Autodesk Inventor part; units mm, degrees
ref_plane "YZ Plane" through (0, 0, 0) normal (1, 0, 0) x (0, 1, 0)
ref_plane "XZ Plane" through (0, 0, 0) normal (0, 1, 0) x (-1, 0, 0)
ref_plane "XY Plane" through (0, 0, 0) normal (0, 0, 1) x (1, 0, 0)
sketch "Sketch1" plane through (0, 0, 0) normal (0, 1, 0) x (-1, 0, 0)
  line L0 (0, 0) -> (105, 0)
  line L1 (105, 0) -> (105, -80)
  line L2 (105, -80) -> (0, -80)
  line L3 (0, -80) -> (0, 0)
  dimension "d0" = 105
  dimension "d1" = 80
extrude "Extrusion1" add sketch "Sketch1" along normal blind 5
sketch "Sketch2" plane through (0, 5, 0) normal (0, 1, 0) x (1, 0, 0)
  line L0 (0, 0) -> (0, 80)
  line L1 (-105, 80) -> (-105, 0)
  line L2 (0, 74) -> (-105, 74)
  line L3 (-105, 74) -> (-105, 7)
  line L4 (-105, 7) -> (0, 7)
  line L5 (0, 7) -> (0, 74)
  line L6 (-105, 0) -> (0, 0)
  line L7 (0, 80) -> (-105, 80)
  line L8 (-60, 7) -> (-60, 0)
  line L9 (-60, 7) -> (-65, 7)
  line L10 (-65, 7) -> (-65, 74)
  line L11 (-65, 74) -> (-60, 74)
  line L12 (-60, 74) -> (-60, 7)
  line L13 (-60, 64) -> (-65, 64)
  line L14 (-65, 64) -> (-65, 17)
  line L15 (-65, 17) -> (-60, 17)
  line L16 (-60, 17) -> (-60, 64)
  line L17 (0, 80) -> (-105, 80)
  line L18 (-105, 80) -> (-105, 0)
  line L19 (-105, 0) -> (0, 0)
  line L20 (0, 0) -> (0, 80)
  point P0 (-62.5, 74)
  point P1 (-62.5, 64)
  point P2 (-62.5, 7)
  point P3 (-62.5, 17)
  dimension "d4" = 7
  dimension "d5" = 6
  dimension "d7" = 45
  dimension "d8" = 5
  dimension "d9" = 10
  dimension "d10" = 10
extrude "Extrusion2" add sketch "Sketch2" along normal blind 25 contours L6 L1 L4 L8 | L2 L1 L7 L0 | L4 L10 L15 L12 | L12 L13 L10 L2
sketch "Sketch3" plane through (0, 30, 0) normal (0, 1, 0) x (1, 0, 0)
  line L0 (-100, 3.5) -> (-5, 3.5)
  line L1 (-5, 3.5) -> (-5, 77)
  line L2 (-5, 77) -> (-100, 77)
  line L3 (-100, 77) -> (-100, 3.5)
  line L4 (0, 80) -> (-105, 80)
  line L5 (-105, 0) -> (-60, 0)
  line L6 (-105, 74) -> (-105, 7)
  line L7 (0, 0) -> (0, 74)
  circle A0 centre (-100, 3.5) radius 1.5
  circle A1 centre (-100, 77) radius 1.5
  dimension "d13" = 3
  dimension "d14" = 3.5
  dimension "d15" = 5
  dimension "d16" = 5
  dimension "d17" = 3
  dimension "d20" = 3
extrude "Extrusion3" cut sketch "Sketch3" against normal blind 10 contours L3 A0 L0 | L0 A0 L3
extrude "Extrusion4" cut sketch "Sketch3" against normal blind 10 contours A1 L2 L3 | L3 L2 A1
pattern_linear "Rectangular Pattern2" count 4 spacing 12 along (1, 0, 0) of "Extrusion3"
pattern_linear "Rectangular Pattern3" count 9 spacing 12 along (1, 0, 0) of "Extrusion4"
sketch "Sketch4" plane through (0, 0, 0) normal (0, -1, 0) x (1, 0, 0)
  line L0 (-10, -12) -> (-80, -12)
  line L1 (-80, -12) -> (-80, -68)
  line L2 (-80, -68) -> (-10, -68)
  line L3 (-10, -68) -> (-10, -12)
  line L4 (0, -80) -> (-105, -80)
  line L5 (0, 0) -> (0, -80)
  line L6 (-80, -60) -> (-10, -68)
  line L7 (-10, -12) -> (-80, -20)
  circle A0 centre (-10, -12) radius 1.5
  circle A1 centre (-10, -68) radius 1.5
  circle A2 centre (-80, -20) radius 1.5
  circle A3 centre (-80, -60) radius 1.5
  point P0 (-80, -40)
  point P1 (-45, -68)
  point P2 (-11.5, -12)
  point P3 (-11.4903, -12.1703)
  dimension "d32" = 70
  dimension "d33" = 40
  dimension "d34" = 45
  dimension "d35" = 56
  dimension "d36" = 40
  dimension "d37" = 20
  dimension "d38" = 3
  dimension "d39" = 3
  dimension "d40" = 3
  dimension "d41" = 3
extrude "Extrusion5" cut sketch "Sketch4" against normal up to next contours L7 A0 L0 | L0 A0 L3 | L3 A0 L7 | A1 L2 L3 | L3 L6 A1 | A2 L1 L7 | L7 L1 A2 | L1 A2 | L2 A1 L6 | A3 L1 L6 | L6 L1 A3 | L1 A3
sketch "Sketch5" plane through (0, 5, 0) normal (0, 1, 0) x (1, 0, 0)
  line L0 (-105, 0) -> (0, 0)
  line L1 (0, 0) -> (-61.099, 0)
  line L2 (-61.099, 0) -> (-61.099, 7)
  line L3 (-61.099, 7) -> (0, 7)
  line L4 (0, 7) -> (0, 0)
  point P0 (-105, 7)
extrude "Extrusion6" add sketch "Sketch5" along normal blind 7.9
sketch "Sketch6" plane through (0, 0, -80) normal (0, 0, -1) x (-1, 0, 0)
  line L0 (97, 22) -> (79, 22)
  line L1 (79, 22) -> (79, 8)
  line L2 (79, 8) -> (97, 8)
  line L3 (97, 8) -> (97, 22)
  line L4 (0, 0) -> (105, 0)
  line L5 (0, 0) -> (0, 30)
  circle A0 centre (97, 8) radius 1.5
  circle A1 centre (97, 22) radius 1.5
  circle A2 centre (79, 22) radius 1.5
  circle A3 centre (79, 8) radius 1.5
  line L6 (105, 0) -> (105, 30)
  point P0 (79, 15)
  point P1 (105, 15)
  dimension "d46" = 15
  dimension "d47" = 14
  dimension "d48" = 18
  dimension "d50" = 3
  dimension "d51" = 3
  dimension "d52" = 3
  dimension "d53" = 3
  dimension "d56" = 8
extrude "Extrusion7" cut sketch "Sketch6" against normal up to surface (6 mm away) contours A2 L1 L0 | L0 L1 A2 | A1 L3 L0 | L0 L3 A1 | A3 L2 L1 | L1 L2 A3 | A0 L2 L3 | L3 L2 A0
sketch "Sketch7" plane through (0, 0, 0) normal (0, -1, 0) x (1, 0, 0)
  line L0 (-32, -27.5) -> (-48, -27.5)
  line L1 (-48, -27.5) -> (-48, -52.5)
  line L2 (-48, -52.5) -> (-32, -52.5)
  line L3 (-32, -52.5) -> (-32, -27.5)
  line L4 (0, 0) -> (0, -80)
  line L5 (-105, 0) -> (0, 0)
  line L6 (-46, -27.5) -> (-46, -52.5)
  line L7 (-44, -27.5) -> (-44, -52.5)
  circle A0 centre (-46, -29.75) radius 1.5
  circle A1 centre (-46, -50.25) radius 1.5
  circle A2 centre (-46, -50.25) radius 3.0104
  circle A3 centre (-46, -29.75) radius 3.0104
  line L8 (-42.9896, -50.25) -> (-42.9896, -52.5)
  line L9 (-42.9896, -29.75) -> (-42.9896, -27.5)
  point P0 (-40, -52.5)
  point P1 (-32, -40)
  point P2 (-46, -40)
  point P3 (-48, -40)
  point P4 (-46, -32.7604)
  point P5 (-46, -47.2396)
  dimension "d57" = 40
  dimension "d58" = 40
  dimension "d59" = 25
  dimension "d60" = 16
  dimension "d62" = 2
  dimension "d63" = 4
  dimension "d64" = 3
  dimension "d65" = 2.25
  dimension "d66" = 2.25
  dimension "d67" = 3
extrude "Extrusion8" cut sketch "Sketch7" against normal up to surface (5 mm away) contours L3 L2 L8 A2 L7 A3 L9 L0 | L7 A2 L6 A3 | A0 L6 | L6 A0 | A1 L6 | L6 A1
sketch "Sketch8" plane through (0, 0, 0) normal (0, -1, 0) x (1, 0, 0)
  line L0 (-32, -53.5) -> (-37, -53.5)
  line L1 (-37, -53.5) -> (-37, -26.5)
  line L2 (-37, -26.5) -> (-32, -26.5)
  line L3 (-32, -26.5) -> (-32, -53.5)
  line L4 (-32, -52.5) -> (-42.9896, -52.5)
  line L5 (-42.9896, -27.5) -> (-32, -27.5)
  line L6 (-32, -27.5) -> (-32, -52.5)
  point P0 (0, 0)
  point P1 (-34.5, -53.5)
  dimension "d70" = 1
  dimension "d71" = 1
  dimension "d72" = 5
extrude "Extrusion9" cut sketch "Sketch8" against normal up to surface (5 mm away)
equation "\"d54\" = d52"
properties part number "sensor_zig"
Check sheet for the modelled part. Datum: model origin and axes. Units: mm. A direction names the side the tool comes from. Give positions to 0.01 mm unless a question says otherwise; leave off trailing zeros. Loops run counter-clockwise (first coordinate to the right, second up) from the corner with the lowest first, then second, coordinate; pieces in that order, holes last. Notation, with made-up numbers: M 47,-27 L 100,-27 A29 cw 100,3 Z; hole C 53,-6 d10. An arc over 180 degrees is marked long. Return JSON: item names as keys, results as strings. Group by question number.
1. Tool access check on faces 1 (the flat face through (-40, 2, -52.5)), 2 (the flat face through (-30, 17, -74)), 3 (the cylindrical face through (-16.195, 25.07, -78.487)), 4 (the flat face through (-52, 0, -39)). Record the directions out of +Z, -Z, +X, -X, +Y, -Y that give a thin tool (end or side, any length) a straight path to the whole face; none if there is none.
2. Go/stop test with flat-tipped pins: pin 1 (1.8 mm diameter, centred on x = -80, z = -60, fed in from +Y); pin 2 (3 mm diameter, centred on x = -56.5, y = 20, fed in from +Z); pin 3 (2.5 mm diameter, centred on x = -88, z = -77, fed in from +Y); pin 4 (10 mm diameter, centred on x = -87, z = -27.5, fed in from +Y). Record where each tip stops, or that it passes through.
3. Mould release check, pull along Y, two halves, no side actions. Record for faces 5 (the cylindrical face through (-80.43, 22.45, -77.04)), 6 (the flat face through (-28, 20, -77)), 7 (the flat face through (-34, 2, -53.5)): released by +Y, released by -Y, zero draft, split by the parting line, or undercut.
4. Thickness scan on L1, parallel to Z at x = -76, y = 27.5; L2, parallel to Z at x = -64, y = 26; L3, parallel to Z at x = -10, y = 2.85. Record the ranges inside material, lowest first.
5. Cross-section at C-C on z = -68. Record the boundary of the cut face in (x, y).
6. Cross-section at B-B on x = -40. Record the boundary of the cut face in (y, z).
7. Cross-section at D-D on x = -97. Record the boundary of the cut face in (y, z), plus the area to 3 significant figures.
8. Cross-section at A-A on y = 18.5. Record the boundary of the cut face in (x, z), plus the area to 4 significant figures.
Return value:
{
 "1": {"face 1": "+Y, -Y", "face 2": "+X, +Y", "face 3": "+Y", "face 4": "+Z, -Z, +X, -X, -Y"},
 "2": {"pin 1": "through", "pin 2": "z = -74", "pin 3": "y = 20", "pin 4": "y = 5"},
 "3": {"face 5": "undercut", "face 6": "released by +Y", "face 7": "zero draft"},
 "4": {"L1": "-80 to -78.5, -75.5 to -74, -7 to -5, -2 to 0", "L2": "-80 to -78.5, -75.5 to -64, -17 to -5, -2 to 0", "L3": "-80 to -69.5, -66.5 to -13.5, -10.5 to 0"},
 "5": {"outline": "M -105,0 L -11.5,0 L -11.5,5 L -60,5 L -60,30 L -65,30 L -65,5 L -105,5 Z; M -8.5,0 L 0,0 L 0,5 L -8.5,5 Z"},
 "6": {"outline": "M 0,-80 L 30,-80 L 30,-78.5 L 20,-78.5 L 20,-75.5 L 30,-75.5 L 30,-74 L 5,-74 L 5,-52.5 L 0,-52.5 Z; M 0,-27.5 L 5,-27.5 L 5,-7 L 12.9,-7 L 12.9,0 L 0,0 Z"},
 "7": {"outline": "M 0,-80 L 6.5,-80 L 6.5,-74 L 5,-74 L 5,-7 L 30,-7 L 30,0 L 0,0 Z; M 9.5,-80 L 20.5,-80 L 20.5,-74 L 9.5,-74 Z; M 23.5,-80 L 30,-80 L 30,-74 L 23.5,-74 Z", "area": "689 mm^2"},
 "8": {"outline": "M -105,-80 L 0,-80 L 0,-74 L -60,-74 L -60,-64 L -65,-64 L -65,-74 L -105,-74 Z; M -105,-7 L -65,-7 L -65,-17 L -60,-17 L -60,0 L -105,0 Z", "area": "1,045 mm^2"}
}
